```python
from build123d import *

# Parameters (mm, degrees)
SKETCH1_W               = 25.4
SKETCH1_H               = 25.4
SKETCH1_W_2             = 22.225
SKETCH1_H_2             = 22.225
BOSS_EXTRUDE1_DEPTH     = 234.95
FILLET1_R               = 2.54
SKETCH2_R               = 2.159
CUT_EXTRUDE1_DEPTH      = 238.560919126
CUT_EXTRUDE2_DEPTH      = 238.560919126
CUT_EXTRUDE2_DEPTH_BACK = 238.560919126
SKETCH3_R               = 1.7
SKETCH3_R_2             = 4.25


with BuildPart() as part:
    # Sketch1 → Boss-Extrude1 (new body)
    with BuildSketch(Plane.XY):
        with Locations((-11.559591837, -1.275183673)):
            Rectangle(SKETCH1_W, SKETCH1_H)
        with Locations((-11.559591837, -1.275183673)):
            Rectangle(SKETCH1_W_2, SKETCH1_H_2, mode=Mode.SUBTRACT)
    extrude(amount=BOSS_EXTRUDE1_DEPTH)

    # Fillet1
    fillet1_edges = [part.edges().sort_by_distance(p)[0] for p in [
        (-24.259591837, 11.424816327, 117.475),
        (1.140408163, 11.424816327, 117.475),
        (1.140408163, -13.975183673, 117.475),
        (-24.259591837, -13.975183673, 117.475),
    ]]
    fillet(fillet1_edges, radius=FILLET1_R)

    # Sketch2 → Cut-Extrude1 (cut, through all)
    with BuildSketch(Plane(origin=(0, 11.424816327, 0), x_dir=(1, 0, 0), z_dir=(0, 1, 0))):
        with Locations(Location((-11.559591837, -12.7, 0), (0, 0, 270))):
            Circle(SKETCH2_R)
        with Locations(Location((-11.559591837, -38.1, 0), (0, 0, 270))):
            Circle(SKETCH2_R)
    extrude(amount=-CUT_EXTRUDE1_DEPTH, mode=Mode.SUBTRACT)

    # Sketch3 → Cut-Extrude2 (cut, two sides: drawn at the far end of the back side and taken through both)
    with BuildSketch(Plane(origin=(0, 11.424816327, 0), x_dir=(1, 0, 0), z_dir=(0, 1, 0)).offset(-CUT_EXTRUDE2_DEPTH_BACK)):
        with Locations(Location((-11.559591837, -207.9, 0), (0, 0, 90))):
            Circle(SKETCH3_R)
        with Locations(Location((-11.559591837, -203.4, 0), (0, 0, 90))):
            Circle(SKETCH3_R)
        with Locations(Location((-11.559591837, -215.9, 0), (0, 0, 90))):
            Circle(SKETCH3_R_2)
        with BuildLine():
            Line((-9.859591837, -223.9), (-9.859591837, -228.4))
            ThreePointArc((-9.859591837, -228.4), (-11.559591837, -230.1), (-13.259591837, -228.4))
            Line((-13.259591837, -228.4), (-13.259591837, -223.9))
            ThreePointArc((-13.259591837, -223.9), (-11.559591837, -222.2), (-9.859591837, -223.9))
        make_face()
    extrude(amount=CUT_EXTRUDE2_DEPTH + CUT_EXTRUDE2_DEPTH_BACK, mode=Mode.SUBTRACT)


solid = part.part
```
Model file for the job. Use its own axes, mm. A direction names the side the tool comes from. Coordinates: 2 decimals unless noted, no trailing zeros. Order: outer loops, then holes, each group sorted by start corner. A loop starts at its lowest first (then second) coordinate and runs counter-clockwise, first axis right, second up. Notation, with made-up numbers: (2.5, 79) -> (44.5, 79) arc R14 ccw to (44.5, 91) -> close; hole circle Ø5 at (-12.75, -18). An arc over 180 degrees is marked (long way). Answer as a JSON object with one key per item and string values. Group by question number.
1) Which spindle directions (+Z, -Z, +X, -X, +Y, -Y) get a long thin tool onto all of the face, cutting with end or side? Do faces 4 (the face through (-12, -12.388, 116)), 5 (the face through (-24.26, -1, 116)). Say none if no direction does.
2) Cut at D-D, the plane z = 215.9. Write the cut outline in (x, y).
3) Cut at B-B, the plane x = -4.75. Write the cut outline in (y, z).
4) Pull direction Z, two halves, no side cores. Call faces 1 (the face through (-12, 9.837, 116)), 2 (the face through (-13.667, 10.642, 37.632)), 3 (the face through (-23, 0, 0)): +Z half, -Z half, draft (parallel to the pull), parting line (faces both ways), or undercut.
5) Cut at C-C, the plane y = -8. Write the cut outline in (x, z), then the cut area to 3 significant figures.
6) Drill centre lines: L1, parallel to X at y = -8.75, z = 211; L2, parallel to Y at x = -8, z = 96; L3, parallel to Y at x = -1, z = 48.5. Where is each one in solid material? Low to high.
7) Cut at A-A, the plane z = 38.1. Write the cut outline in (x, y), then the cut area to 3 significant figures.
8) Flat gauge pins, fed straight in: pin 1 (0.5 mm diameter, centred on y = -13, z = 226, fed in from -X); pin 2 (1.7 mm diameter, centred on y = 10.5, z = 226, fed in from +X). Where does each tip first touch, or does it go through?
Check values:
{
 "1": {"face 4": "+Z, -Z", "face 5": "+Z, -Z, -X, +Y, -Y"},
 "2": {"outline": "(-24.26, -11.44) arc R2.54 ccw to (-21.72, -13.98) -> (-15.81, -13.98) -> (-15.81, -12.39) -> (-22.67, -12.39) -> (-22.67, 9.84) -> (-15.81, 9.84) -> (-15.81, 11.42) -> (-21.72, 11.42) arc R2.54 ccw to (-24.26, 8.88) -> close; (-7.31, -13.98) -> (-1.4, -13.98) arc R2.54 ccw to (1.14, -11.44) -> (1.14, 8.88) arc R2.54 ccw to (-1.4, 11.42) -> (-7.31, 11.42) -> (-7.31, 9.84) -> (-0.45, 9.84) -> (-0.45, -12.39) -> (-7.31, -12.39) -> close"},
 "3": {"outline": "(-13.98, 0) -> (-12.39, 0) -> (-12.39, 234.95) -> (-13.98, 234.95) -> close; (9.84, 0) -> (11.42, 0) -> (11.42, 234.95) -> (9.84, 234.95) -> close"},
 "4": {"face 1": "draft", "face 2": "undercut", "face 3": "-Z half"},
 "5": {"outline": "(-24.26, 0) -> (-22.67, 0) -> (-22.67, 234.95) -> (-24.26, 234.95) -> close; (-0.45, 0) -> (1.14, 0) -> (1.14, 234.95) -> (-0.45, 234.95) -> close", "area": "746 mm²"},
 "6": {"L1": "x = -24.26 to -22.67, -0.45 to 1.14", "L2": "y = -13.98 to -12.39, 9.84 to 11.42", "L3": "y = -13.94 to -12.39, 9.84 to 11.39"},
 "7": {"outline": "(-24.26, -11.44) arc R2.54 ccw to (-21.72, -13.98) -> (-13.72, -13.98) -> (-13.72, -12.39) -> (-22.67, -12.39) -> (-22.67, 9.84) -> (-13.72, 9.84) -> (-13.72, 11.42) -> (-21.72, 11.42) arc R2.54 ccw to (-24.26, 8.88) -> close; (-9.4, -13.98) -> (-1.4, -13.98) arc R2.54 ccw to (1.14, -11.44) -> (1.14, 8.88) arc R2.54 ccw to (-1.4, 11.42) -> (-9.4, 11.42) -> (-9.4, 9.84) -> (-0.45, 9.84) -> (-0.45, -12.39) -> (-9.4, -12.39) -> close", "area": "132 mm²"},
 "8": {"pin 1": "stops at x = -23.89", "pin 2": "stops at x = 1.02"}
}
